For this review, take the finished solid that the model builds, in its own axes (mm). Face numbers are marked on the shaded views. A direction names the side the tool comes from. Give positions to 0.01 mm unless a question says otherwise; leave off trailing zeros. Order: outer loops, then holes, each group sorted by start corner. A loop starts at its lowest first (then second) coordinate and runs counter-clockwise, first axis right, second up. Notation, with made-up numbers: (66, 24) - (103, 24) arc R16 cw to (103, 48) - close; hole circle Ø1 at (81, -15). An arc over 180 degrees is marked (long way). One line per item, written item: value.
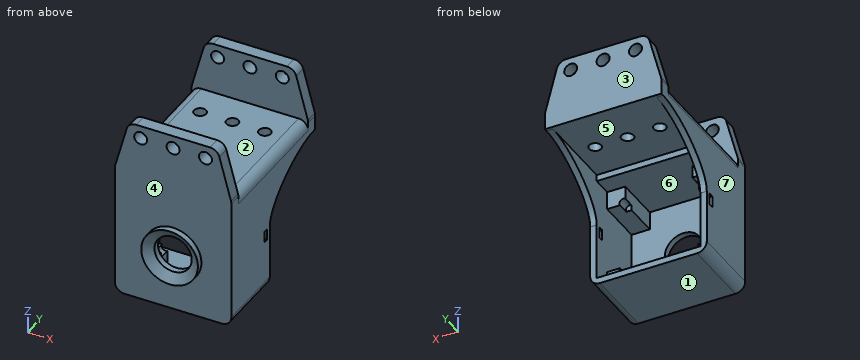
```python
from build123d import *

# Parameters (mm, degrees)
SKETCH1_W           = 40.64
SKETCH1_H           = 40.64
BOSS_EXTRUDE1_DEPTH = 25.4
SHELL1_T            = 2.54
SKETCH2_W           = 7.112
SKETCH2_H           = 7.112
BOSS_EXTRUDE2_DEPTH = 17.78
BOSS_EXTRUDE3_DEPTH = 60.96
SKETCH5_W           = 20.32
SKETCH5_H           = 50.8
CUT_EXTRUDE1_DEPTH  = 90.198854813
SKETCH6_R           = 2.54
CUT_EXTRUDE2_DEPTH  = 82.804169209
FILLET1_R           = 3.81
SKETCH10_R          = 1.524
CUT_EXTRUDE4_DEPTH  = 4.572
CIRPATTERN1_COUNT   = 4
SKETCH11_R          = 7.3025
CUT_EXTRUDE5_DEPTH  = 80.929324406
RIB1_START          = -2.54
RIB1_DEPTH          = 2.54
SKETCH19_R          = 2.38125
CUT_EXTRUDE6_DEPTH  = 78.625990598
SKETCH20_W          = 2.032
SKETCH20_H          = 4.445


with BuildPart() as part:
    # Sketch1 → Boss-Extrude1 (new body)
    with BuildSketch(Plane(origin=(0, 0, 0), x_dir=(1, 0, 0), z_dir=(0, 1, 0))):
        Rectangle(SKETCH1_W, SKETCH1_H)
    extrude(amount=BOSS_EXTRUDE1_DEPTH)

    # Shell1
    shell1_openings = [part.faces().sort_by_distance(p)[0] for p in [
        (0, 25.4, 0),
    ]]
    offset(amount=SHELL1_T, openings=shell1_openings, kind=Kind.INTERSECTION)

    # Sketch2 → Boss-Extrude2 (add)
    with BuildSketch(Plane(origin=(0, 0, 0), x_dir=(1, 0, 0), z_dir=(0, 1, 0))):
        with Locations((-16.764, 16.764)):
            Rectangle(SKETCH2_W, SKETCH2_H)
    boss_extrude2 = extrude(amount=BOSS_EXTRUDE2_DEPTH)

    # Sketch3 → Boss-Extrude3 (add)
    with BuildSketch(Plane.XZ.offset(2.54)):
        with BuildLine():
            Line((-22.730177398, 29.694504546), (-17.41527241, 49.53))
            Line((-17.41527241, 49.53), (17.41527241, 49.53))
            Line((17.41527241, 49.53), (22.730177398, 29.694504546))
            ThreePointArc((22.730177398, 29.694504546), (22.827404922, 29.205708777), (22.86, 28.708403984))
            Line((22.86, 28.708403984), (22.86, 22.86))
            Line((22.86, 22.86), (-22.86, 22.86))
            Line((-22.86, 22.86), (-22.86, 28.708403984))
            ThreePointArc((-22.86, 28.708403984), (-22.827404922, 29.205708777), (-22.730177398, 29.694504546))
        make_face()
    extrude(amount=-BOSS_EXTRUDE3_DEPTH)

    # Sketch5 → Cut-Extrude1 (cut, through all)
    with BuildSketch(Plane.ZY.offset(22.86)):
        with Locations((39.37, 27.94)):
            Rectangle(SKETCH5_W, SKETCH5_H)
    extrude(amount=-CUT_EXTRUDE1_DEPTH, mode=Mode.SUBTRACT)

    # Sketch6 → Cut-Extrude2 (cut, through all)
    with BuildSketch(Plane(origin=(0, 58.42, 0), x_dir=(1, 0, 0), z_dir=(0, 1, 0))):
        with Locations(Location((-12.7, -44.45, 0), (0, 0, 270))):
            Circle(SKETCH6_R)
        with Locations(Location((0, -44.45, 0), (0, 0, 270))):
            Circle(SKETCH6_R)
        with Locations(Location((12.7, -44.45, 0), (0, 0, 270))):
            Circle(SKETCH6_R)
    extrude(amount=-CUT_EXTRUDE2_DEPTH, mode=Mode.SUBTRACT)

    # Fillet1
    # the kernel refuses this fillet: 3.81 mm, written as the material it takes off along each edge
    with BuildSketch(Plane(origin=(-17.41527241, 46.03121044, 49.53), x_dir=(-0.25881904510252424, 0, -0.9659258262890673), z_dir=(0, 1, 0)), Plane(origin=(17.41527241, 46.03121044, 49.53), x_dir=(-1, 0, 0), z_dir=(0, 1, 0)), Plane(origin=(-17.41527241, -9.84878956, 49.53), x_dir=(-0.25881904510252424, 0, -0.9659258262890673), z_dir=(0, 1, 0)), Plane(origin=(17.41527241, -9.84878956, 49.53), x_dir=(-1, 0, 0), z_dir=(0, 1, 0))) as fillet1_piece_1:
        with BuildLine():
            CenterArc((FILLET1_R * 0.767326987979, -FILLET1_R), FILLET1_R, 90, 75)
            Line((-FILLET1_R * 0.19859883831, -FILLET1_R * 0.741180954897), (0, 0))
            Line((0, 0), (FILLET1_R * 0.767326987979, 0))
        make_face()
    extrude(amount=19.697579121, mode=Mode.SUBTRACT)
    with BuildSketch(Plane(origin=(-22.826837491, 53.34, 29.21), x_dir=(-0.008703740786851863, 0, -0.999962121730776), z_dir=(0, -1, 0))) as fillet1_piece_2:
        with BuildLine():
            CenterArc((3.776983069, 3.809855684), FILLET1_R, 180.49869391, 90)
            Line((-0.032872615, 3.776694431), (-0.413858183, 3.773378306))
            Line((-0.413858183, 3.773378306), (-0.380985568, -0.003316125))
            Line((-0.380985568, -0.003316125), (-0.04687044, -0.378106019))
            ThreePointArc((-0.04687044, -0.378106019), (0.505181779, -0.409781059), (3.813460447, -0.380985568))
            Line((3.813460447, -0.380985568), (3.810144322, 0))
        make_face()
    extrude(amount=50.8, mode=Mode.SUBTRACT)
    with BuildSketch(Plane(origin=(22.826837491, 53.34, 29.21), x_dir=(0.008703740786853719, 0, -0.999962121730776), z_dir=(0, -1, 0))) as fillet1_piece_3:
        with BuildLine():
            CenterArc((3.776983069, -3.809855684), FILLET1_R, 89.50130609, 90)
            Line((-0.032872615, -3.776694431), (-0.413858183, -3.773378306))
            Line((-0.413858183, -3.773378306), (-0.380985568, 0.003316125))
            Line((-0.380985568, 0.003316125), (-0.04687044, 0.378106019))
            ThreePointArc((-0.04687044, 0.378106019), (0.505181779, 0.409781059), (3.813460447, 0.380985568))
            Line((3.813460447, 0.380985568), (3.810144322, 0))
        make_face()
    extrude(amount=50.8, mode=Mode.SUBTRACT)
    with BuildSketch(Plane(origin=(-22.86, -12.065, -22.86), x_dir=(1, 0, 0), z_dir=(0, 1, 0))) as fillet1_piece_4:
        with BuildLine():
            CenterArc((FILLET1_R, -FILLET1_R), FILLET1_R, 90, 90)
            Line((0, -FILLET1_R), (0, 0))
            Line((0, 0), (FILLET1_R, 0))
        make_face()
    extrude(amount=46.99, mode=Mode.SUBTRACT)
    with BuildSketch(Plane(origin=(22.86, -12.065, -22.86), x_dir=(-1, 0, 0), z_dir=(0, 1, 0))) as fillet1_piece_5:
        with BuildLine():
            CenterArc((FILLET1_R, FILLET1_R), FILLET1_R, 180, 90)
            Line((0, FILLET1_R), (0, 0))
            Line((0, 0), (FILLET1_R, 0))
        make_face()
    extrude(amount=46.99, mode=Mode.SUBTRACT)

    # Sketch10 → Cut-Extrude4 (cut)
    with BuildSketch(Plane.XZ.offset(-13.208)):
        with Locations((-13.97, -13.97)):
            Circle(SKETCH10_R)
    cut_extrude4 = extrude(amount=-CUT_EXTRUDE4_DEPTH, mode=Mode.SUBTRACT)

    # CirPattern1: Boss-Extrude2, Cut-Extrude4 ×4 about axis
    cirpattern1_axis = Axis((0, 0, 0), (0, 1, 0))
    add([boss_extrude2.rotate(cirpattern1_axis, i * 360 / CIRPATTERN1_COUNT) for i in range(1, CIRPATTERN1_COUNT)])
    add([cut_extrude4.rotate(cirpattern1_axis, i * 360 / CIRPATTERN1_COUNT) for i in range(1, CIRPATTERN1_COUNT)], mode=Mode.SUBTRACT)

    # Sketch11 → Cut-Extrude5 (cut, through all)
    with BuildSketch(Plane(origin=(0, 0, 0), x_dir=(1, 0, 0), z_dir=(0, 1, 0))):
        with Locations(Location((0, 0, 0), (0, 0, 270))):
            Circle(SKETCH11_R)
    extrude(amount=-CUT_EXTRUDE5_DEPTH, mode=Mode.SUBTRACT)

    # Sketch12 → Revolve1 (revolve)
    with BuildSketch(Plane.XY, mode=Mode.PRIVATE) as revolve1_sk:
        Polygon((-11.1125, -2.54), (-11.1125, -5.08), (-7.3025, -2.54), align=None)
    revolve(revolve1_sk.sketch.rotate(Axis((0, 12.66825, 0), (0, -1, 0)), 270), axis=Axis((0, 12.66825, 0), (0, -1, 0)))

    # Rib1: read off the stored shape, not the designer's step
    # Rib1 outline → Rib1 (add)
    with BuildSketch(Plane.ZY.offset(22.86).offset(RIB1_START)):
        with BuildLine():
            add(Edge.make_bspline(
                [(1.905, 25.4), (11.363397975, 25.4), (22.86, 44.45), (22.86, 57.15)],
                knots=[0, 0, 0, 0, 1, 1, 1, 1], degree=3))
            Line((1.905, 25.4), (22.86, 25.4))
            Line((22.86, 25.4), (22.86, 57.15))
        make_face()
    rib1 = extrude(amount=RIB1_DEPTH)

    # Mirror2: Rib1 across plane
    add(rib1.mirror(Plane(origin=(0, 0, 0), x_dir=(0, 0, 1), z_dir=(1, 0, 0))))

    # Sketch19 → Cut-Extrude6 (cut, through all)
    with BuildSketch(Plane(origin=(0, 0, 22.86), x_dir=(-1, 0, 0), z_dir=(0, 0, -1))):
        with Locations((-12.7, 40.64)):
            Circle(SKETCH19_R)
        with Locations((12.7, 40.64)):
            Circle(SKETCH19_R)
        with Locations((0, 40.64)):
            Circle(SKETCH19_R)
    extrude(amount=-CUT_EXTRUDE6_DEPTH, mode=Mode.SUBTRACT)

    # Cut-Sweep1: sweep along a path in Sketch21
    with BuildLine() as cut_sweep1_path:  # in the path sketch's own coordinates; laid on its plane below (add() does not lay a ready-made edge on the line's plane)
        Line((-22.86, 22.4155), (-19.05, 22.4155))
        add(Edge.make_bspline(
            [(-19.05, 22.4155), (-16.933333333, 22.4155), (-15.24, 23.791333333), (-15.24, 25.273)],
            knots=[0, 0, 0, 0, 1, 1, 1, 1], degree=3))
    # Sketch20 → Cut-Sweep1 (sweep, cut)
    with BuildSketch(Plane(origin=(0, 25.273, 0), x_dir=(1, 0, 0), z_dir=(0, 1, 0))):
        with Locations((-15.24, 0)):
            Rectangle(SKETCH20_W, SKETCH20_H)
    cut_sweep1 = sweep(path=Plane.XY * cut_sweep1_path.line, mode=Mode.SUBTRACT)

    # Mirror4: Cut-Sweep1 across plane
    add(cut_sweep1.mirror(Plane(origin=(0, 0, 0), x_dir=(0, 0, 1), z_dir=(1, 0, 0))), mode=Mode.SUBTRACT)


solid = part.part
```
(1) Wall thickness on line 1 (Z direction, x = -10.5, y = 4); line 2 (Y direction, x = -12.7, z = 27.5); line 3 (X direction, y = 4, z = -19): over which ranges is each line inside the solid? List them lowest first. Write a range as from..to.
Answers below:
line 1: z = -22.86..-20.32, 20.32..29.21
line 2: y = -2.54..38.26, 43.02..58.42
line 3: x = -22.86..-13.21, 13.21..22.86
(2) Take a section at D-D (z = -18). Write out the cut boundary in (x, y), then the cut area to 3 significant figures.
Answers below:
outline: (-22.86, -2.54) - (22.86, -2.54) - (22.86, 25.4) - (20.32, 25.4) - (20.32, 17.78) - (13.21, 17.78) - (13.21, 0) - (-13.21, 0) - (-13.21, 17.78) - (-20.32, 17.78) - (-20.32, 25.4) - (-22.86, 25.4) - close
area: 498 mm^2
(3) Draft analysis for pull direction Y (two halves, no side actions). For the marked faces 1, 2 and 3, state which applies: pulls with the +Y half, pulls with the -Y half, needs draft (parallel to the pull), parting line crosses it, or undercut.
Answers below:
face 1: needs draft
face 2: undercut
face 3: pulls with the +Y half
(4) Machinability: for the marked faces 4, 5, 6 and 7, which of the approach directions +Z, -Z, +X, -X, +Y, -Y give a long, thin tool a straight path to every point of the face, cutting with its end or side? Answer none if there is none.
Answers below:
face 4: -Y
face 5: -Z, +Y
face 6: +Y
face 7: +Z, -Z, -X, +Y, -Y
(5) For P1, Ø12, axis at x = 4, z = 16, coming from the +Y side; P2, Ø0.8, axis at x = -21.5, z = 0, coming from the -Y side; P3, Ø0.7, axis at x = -14, z = -15, coming from the +Y side; P4, Ø8, axis at x = 0, z = 44.45, coming from the +Y side, all flat-tipped, find the tip position at first contact; note any pin that passes through.
Answers below:
P1: stops at y = 25.4
P2: stops at y = -2.54
P3: stops at y = 13.21
P4: stops at y = 58.42
(6) Take a section at A-A (z = 0). Write out the cut boundary in (x, y), then the cut area to 3 significant figures.
Answers below:
outline: (-22.86, -2.54) - (-11.11, -2.54) - (-11.11, -5.08) - (-7.3, -2.54) - (-7.3, 0) - (-20.32, 0) - (-20.32, 21.4) - (-22.86, 21.4) - close; (-22.86, 23.43) - (-20.32, 23.43) - (-20.32, 25.4) - (-22.86, 25.4) - close; (7.3, -2.54) - (11.11, -5.08) - (11.11, -2.54) - (22.86, -2.54) - (22.86, 21.4) - (20.32, 21.4) - (20.32, 0) - (7.3, 0) - close; (20.32, 23.43) - (22.86, 23.43) - (22.86, 25.4) - (20.32, 25.4) - close
area: 207 mm^2
(7) Take a section at C-C (z = 44.45). Give the number of separate pieces and of enclosed holes in the cut face, then the cut area to 3 significant figures.
Answers below:
separate pieces: 8
enclosed holes: 0
area: 227 mm^2
(8) Take a section at B-B (y = 11.5). Write out the cut boundary in (x, z).
Answers below:
outline: (-22.86, -19.05) arc R3.81 ccw to (-19.05, -22.86) - (19.05, -22.86) arc R3.81 ccw to (22.86, -19.05) - (22.86, 25.4) arc R3.81 ccw to (19.05, 29.21) - (-19.05, 29.21) arc R3.81 ccw to (-22.86, 25.4) - close; hole (-20.32, -13.21) - (-13.21, -13.21) - (-13.21, -20.32) - (13.21, -20.32) - (13.21, -13.21) - (20.32, -13.21) - (20.32, 13.21) - (13.21, 13.21) - (13.21, 20.32) - (-13.21, 20.32) - (-13.21, 13.21) - (-20.32, 13.21) - close
